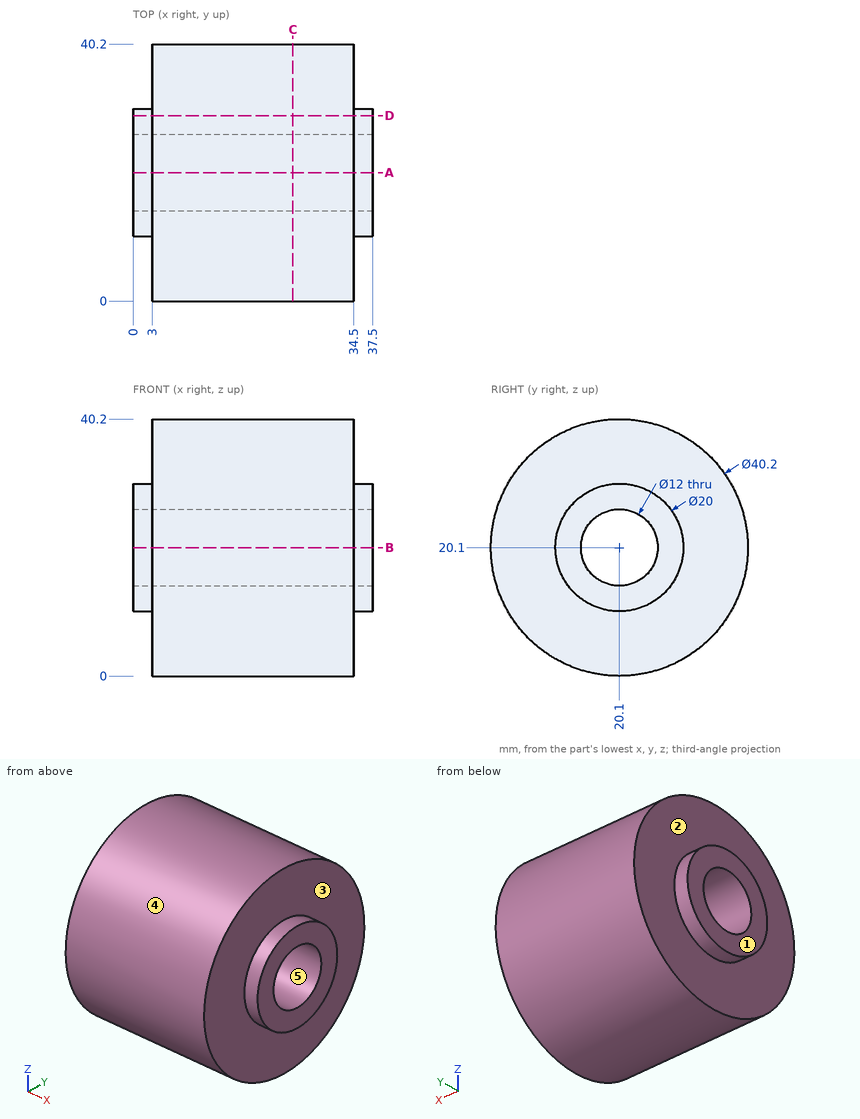
Answer from the drawing. Dimensions are ordinates in mm from the lowest x, y and z of the part. A direction names the side the tool comes from. Coordinates: 2 decimals unless noted, no trailing zeros. Write each loop counter-clockwise with the first axis right and the second up, starting at its lowest first coordinate (ties: lowest second). Pieces come first, ordered by that corner, then holes. Notation, with made-up numbers: M 24.5,58 L 56.5,58 A20 ccw 56.5,84 Z; hole C -12.5,-15.75 d9. An arc over 180 degrees is marked long. Write item = value, one per line.
1. Determine the mould class of the marked faces 3, 4 and 5 for opening direction Y: released by +Y, released by -Y, zero draft, split by the parting line, or undercut.
Solution:
face_3 = zero draft
face_4 = split by the parting line
face_5 = undercut
2. The part is cut by section C-C (x = 25). Determine the outline of the cut face in (y, z), then the cut area to 3 significant figures.
Solution:
outline = C 20.1,20.1 d40.2; hole C 20.1,20.1 d12
area = 1,160 mm2
3. The part is cut by section D-D (y = 29). Determine the outline of the cut face in (x, z).
Solution:
outline = M 0,15.54 L 3,15.54 L 3,2.08 L 34.5,2.08 L 34.5,15.54 L 37.5,15.54 L 37.5,24.66 L 34.5,24.66 L 34.5,38.12 L 3,38.12 L 3,24.66 L 0,24.66 Z
4. For the marked faces 1 and 2, determine the directions among +Z, -Z, +X, -X, +Y, -Y from which every point of the face is accessible in a straight line to the end or side of a thin tool.
Solution:
face_1 = +Z, -Z, -X, +Y, -Y
face_2 = -X
5. Straight lines are drawn through the part: line 1 (Y direction, x = 8, z = 20); line 2 (Y direction, x = 22.5, z = 16). For each, find the intervals that lie inside material, in ascending order. Write a range as from..to.
Solution:
line_1 = 0..14.1, 26.1..40.2
line_2 = 0.42..15.72, 24.48..39.78
6. Flat-ended cylindrical pins translate along their axes: pin 1 (2 mm diameter, centred on y = 33.5, z = 13, fed in from +X); pin 2 (3 mm diameter, centred on x = 25, z = 8.5, fed in from +Y); pin 3 (5 mm diameter, centred on x = 24.5, z = 10, fed in from +Y). Find the tip coordinate at first contact, or state that the pin passes through.
Solution:
pin_1 = 34.5
pin_2 = 37.48
pin_3 = 38.71
7. The part is cut by section A-A (y = 20.1). Determine the outline of the cut face in (x, z), then the cut area to 3 significant figures.
Solution:
outline = M 0,10.1 L 3,10.1 L 3,0 L 34.5,0 L 34.5,10.1 L 37.5,10.1 L 37.5,14.1 L 0,14.1 Z; M 0,26.1 L 37.5,26.1 L 37.5,30.1 L 34.5,30.1 L 34.5,40.2 L 3,40.2 L 3,30.1 L 0,30.1 Z
area = 936 mm2
